Input: part model. Units: mm. Frame: model coordinates. Give positions to 0.01 mm unless a question says otherwise; leave off trailing zeros. Write each loop counter-clockwise with the first axis right and the second up, starting at its lowest first coordinate (ties: lowest second). Pieces come first, ordered by that corner, then holes.
```python
from build123d import *

# Parameters (mm, degrees)
ESBO_O1_R                  = 8
ESBO_O1_R_2                = 7.25
RESSALTO_EXTRUS_O1_DEPTH   = 300
CORTE_EXTRUS_O1_DEPTH      = 300
CORTE_EXTRUS_O1_DEPTH_BACK = 300
ESBO_O2_R                  = 1.75
CUT_EXTRUDE1_REACH         = 302.213
CUT_EXTRUDE1_END_RADIUS    = 8
SKETCH2_R                  = 3.5


with BuildPart() as part:
    # Esboço1 → Ressalto-extrusão1 (new body)
    with BuildSketch(Plane.XY):
        Circle(ESBO_O1_R)
        Circle(ESBO_O1_R_2, mode=Mode.SUBTRACT)
    extrude(amount=RESSALTO_EXTRUS_O1_DEPTH)

    # Esboço2 → Corte-extrusão1 (cut, two sides: drawn at the far end of the back side and taken through both)
    with BuildSketch(Plane(origin=(0, 0, 0), x_dir=(0, 0, -1), z_dir=(1, 0, 0)).offset(-CORTE_EXTRUS_O1_DEPTH_BACK)):
        with Locations(Location((-293, 0, 0), (0, 0, 180))):
            Circle(ESBO_O2_R)
        with Locations(Location((-283, 0, 0), (0, 0, 180))):
            Circle(ESBO_O2_R)
    extrude(amount=CORTE_EXTRUS_O1_DEPTH + CORTE_EXTRUS_O1_DEPTH_BACK, mode=Mode.SUBTRACT)

    # Cut-Extrude1: up to this cylinder (the profile starts inside it)
    cut_extrude1_end = Plane(origin=(0, 0, 147), z_dir=(0, 0, -1)) * Cylinder(CUT_EXTRUDE1_END_RADIUS, 621.426, mode=Mode.PRIVATE)
    # Sketch2 → Cut-Extrude1 (cut, up to the surface)
    with BuildSketch(Plane(origin=(0, 0, 0), x_dir=(1, 0, 0), z_dir=(0, 1, 0)), mode=Mode.PRIVATE) as cut_extrude1_sk1:
        with Locations(Location((0, -147, 0), (0, 0, 270))):
            Circle(SKETCH2_R)
    cut_extrude1_tool1 = extrude(cut_extrude1_sk1.sketch, amount=-CUT_EXTRUDE1_REACH, mode=Mode.PRIVATE) & cut_extrude1_end
    add(cut_extrude1_tool1.solids().sort_by_distance((0, 0, 147))[0], mode=Mode.SUBTRACT)


solid = part.part
```
Q1. Section C-C, the plane z = 147. Return the cut outline in (x, y).
Q2. Material intervals for line 1 along X through (y, z) = (0, 74); line 2 along X through (y, z) = (-4.5, 266.5); line 3 along Y through (x, z) = (2.25, 124), sorted ascending.
Q3. Section B-B, the plane z = 193. Return the cut outline in (x, y).
Q4. Pin query (flat end, axial travel): pin 1 (8 mm diameter, centred on x = -6.5, z = 100, fed in from +Y). Return the tip coordinate at first contact, or that it passes through.
Q5. Mould query, pull axis Y, two halves, no side actions, for faces 1 (the cylindrical face through (4.301, 6.746, 147.9)), 2 (the cylindrical face through (-0.94, 7.19, 147.9)). Classes: +Y half, -Y half, draft (parallel to the pull), parting line (faces both ways), or undercut.
Q6. Section A-A, the plane x = 0. Return the cut outline in (y, z), then the cut area to 3 significant figures.
Solutions:
1. outline: (-3.5, -7.19) - (-3.5, -6.35) arc R7.25 cw (long way) to (3.5, -6.35) - (3.5, -7.19) arc R8 ccw (long way) to start
2. line 1: x = -8 to -7.25, 7.25 to 8
2. line 2: x = -6.61 to -5.68, 5.68 to 6.61
2. line 3: y = -7.68 to -6.89, 6.89 to 7.68
3. outline: circle Ø16 at (0, 0); hole circle Ø14.5 at (0, 0)
4. pin 1: stops at y = 7.6
5. face 1: parting line
5. face 2: undercut
6. outline: (-8, 0) - (-7.25, 0) - (-7.25, 143.5) - (-8, 143.5) - close; (-8, 150.5) - (-7.25, 150.5) - (-7.25, 300) - (-8, 300) - close; (7.25, 0) - (8, 0) - (8, 300) - (7.25, 300) - close
6. area: 445 mm2
